For this review, take the finished solid that the model builds, in its own axes (mm). A direction names the side the tool comes from. Round coordinates to 2 decimals unless told otherwise and drop trailing zeros. Loops run counter-clockwise (first coordinate to the right, second up) from the corner with the lowest first, then second, coordinate; pieces in that order, holes last.
```python
from build123d import *

# Parameters (mm, degrees)
SKETCH1_R           = 18.2
BOSS_EXTRUDE1_DEPTH = 22
SKETCH5_R           = 18.2
SKETCH5_R_2         = 4
BOSS_EXTRUDE4_DEPTH = 18
CUT_EXTRUDE1_DEPTH  = 48.56553374
SKETCH7_R           = 3.1
CUT_EXTRUDE2_DEPTH  = 18


with BuildPart() as part:
    # Sketch1 → Boss-Extrude1 (new body)
    with BuildSketch(Plane(origin=(0, 0, 0), x_dir=(1, 0, 0), z_dir=(0, 1, 0))):
        with Locations(Location((0, 0, 0), (0, 0, 270))):
            Circle(SKETCH1_R)
        with BuildLine():
            Line((2, 7.3), (2, 5.8685603))
            ThreePointArc((2, 5.8685603), (5.041825066, 3.608323711), (6.2, 0))
            ThreePointArc((6.2, 0), (-3.608323711, -5.041825066), (-2, 5.8685603))
            Line((-2, 5.8685603), (-2, 7.3))
            Line((-2, 7.3), (2, 7.3))
        make_face(mode=Mode.SUBTRACT)
    extrude(amount=BOSS_EXTRUDE1_DEPTH)

    # Sketch5 → Boss-Extrude4 (add)
    with BuildSketch(Plane(origin=(0, 22, 0), x_dir=(1, 0, 0), z_dir=(0, 1, 0))):
        with Locations(Location((0, 0, 0), (0, 0, 270))):
            Circle(SKETCH5_R)
        with Locations(Location((0, 0, 0), (0, 0, 270))):
            Circle(SKETCH5_R_2, mode=Mode.SUBTRACT)
    extrude(amount=BOSS_EXTRUDE4_DEPTH)

    # Sketch6 → Cut-Extrude1 (cut, through all)
    with BuildSketch(Plane.XZ):
        Polygon((17.499714283, 100.15185494), (17.499714283, 5), (17.499714283, -5), (17.499714283, -100.15185494), (207.803424163, -100.15185494), (207.803424163, 100.15185494), align=None)
    extrude(amount=-CUT_EXTRUDE1_DEPTH, mode=Mode.SUBTRACT)

    # Sketch7 → Cut-Extrude2 (cut)
    with BuildSketch(Plane(origin=(17.499714283, 0, 0), x_dir=(0, 0, -1), z_dir=(1, 0, 0))):
        with Locations((0, 10)):
            Circle(SKETCH7_R)
        with Locations((0, 32)):
            Circle(SKETCH7_R)
    extrude(amount=-CUT_EXTRUDE2_DEPTH, mode=Mode.SUBTRACT)


solid = part.part
```
(1) For faces 4 (the flat face through (4.2, 22, -0.6)), 5 (the cylindrical face through (10.1, 32.1, 3.1)), 6 (the flat face through (0, 0, 8)), list the 3-axis set-ups (+Z, -Z, +X, -X, +Y, -Y) from which the entire face can be reached by the end or side of a thin tool; tool diameter is ignored.
(2) Add section D-D (y = 32). Give the boundary of the cut face in (x, z), plus the area to 3 significant figures.
(3) For L1, parallel to Y at x = 11, z = 0; L2, parallel to Z at x = 0, y = 14.5; L3, parallel to Y at x = 5.5, z = 0, list the stretches that pass through material, from the lowest coordinate up.
(4) Add section A-A (z = 2). Give the boundary of the cut face in (x, y).
(5) Add section B-B (x = 0). Give the boundary of the cut face in (y, z).
(6) Insertion check: pin 1 Ø4 at (x, y) = (8.5, 29) entering from -Z; pin 2 Ø2 at (x, y) = (9, 22) entering from +Z; pin 3 Ø10 at (y, z) = (32, 0) entering from -X. Each pin has a flat end and moves straight along its axis. Give the tip position at first contact, or say it passes through.
(7) Add section C-C (y = 15). Give the boundary of the cut face in (x, z).
(8) The part is to be moulded in two halves that separate along Z. For faces 1 (the flat face through (-0.1, 40, -4.3)), 2 (the flat face through (2, 11, -7)), 3 (the cylindrical face through (-18.185, 19.72, -0.729)), say which applies: pulls with the +Z half, pulls with the -Z half, needs draft (parallel to the pull), parting line crosses it, or undercut.
Outcome:
1. face 4: -Y
1. face 5: +X
1. face 6: +Z, -Z, +X, -X, -Y
2. outline: (2.53, -3.1) arc R4 cw (long way) to (2.53, 3.1) - (17.5, 3.1) - (17.5, 5) arc R18.2 ccw (long way) to (17.5, -5) - (17.5, -3.1) - close
2. area: 899 mm2
3. L1: y = 0 to 6.9, 13.1 to 28.9, 35.1 to 40
3. L2: z = -18.2 to -7.3, 6.2 to 18.2
3. L3: y = 22 to 28.9, 35.1 to 40
4. outline: (-18.09, 0) - (-5.87, 0) - (-5.87, 22) - (-3.46, 22) - (-3.46, 40) - (-18.09, 40) - close; (3.46, 22) - (5.87, 22) - (5.87, 12.37) - (17.5, 12.37) - (17.5, 29.63) - (3.46, 29.63) - close; (3.46, 34.37) - (17.5, 34.37) - (17.5, 40) - (3.46, 40) - close; (5.87, 0) - (17.5, 0) - (17.5, 7.63) - (5.87, 7.63) - close
5. outline: (0, -18.2) - (40, -18.2) - (40, -4) - (22, -4) - (22, -7.3) - (0, -7.3) - close; (0, 6.2) - (22, 6.2) - (22, 4) - (40, 4) - (40, 18.2) - (0, 18.2) - close
6. pin 1: stops at z = -17
6. pin 2: stops at z = 16.35
6. pin 3: stops at x = -18.2
7. outline: (17.5, -5) - (17.5, 5) arc R18.2 ccw (long way) to start; hole (-2, -7.3) - (2, -7.3) - (2, -5.87) arc R6.2 ccw (long way) to (-2, -5.87) - close
8. face 1: needs draft
8. face 2: undercut
8. face 3: parting line crosses it
